Source: three-view drawing plus pictorial views. Frame: mm from the lowest corner of the part. Coordinates: 2 decimals unless noted, no trailing zeros. Write each loop counter-clockwise with the first axis right and the second up, starting at its lowest first coordinate (ties: lowest second). Pieces come first, ordered by that corner, then holes. Notation, with made-up numbers: (0.5, 70.25) - (8.5, 70.25) arc R33 ccw to (8.5, 104.25) - close; hole circle Ø7 at (-13.75, 80). An arc over 180 degrees is marked (long way). One line per item, written item: value.
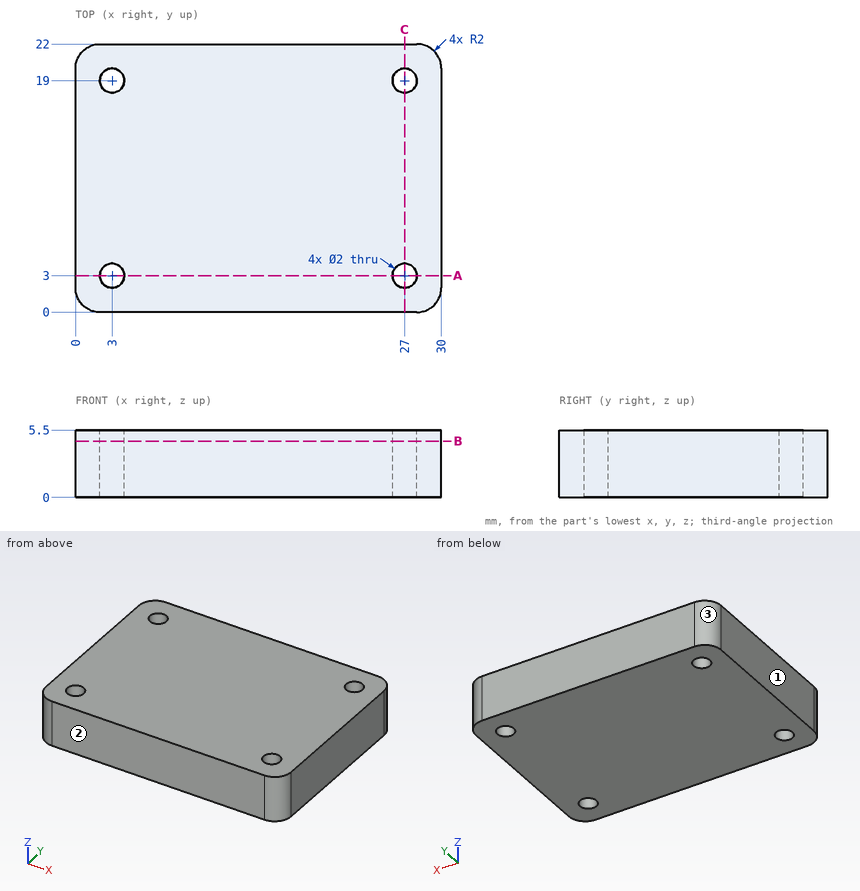
1) Section query B-B on z = 4.6. Output: boundary loops of the cut face in (x, y).
Values found:
outline: (0, 2) arc R2 ccw to (2, 0) - (28, 0) arc R2 ccw to (30, 2) - (30, 20) arc R2 ccw to (28, 22) - (2, 22) arc R2 ccw to (0, 20) - close; hole circle Ø2 at (3, 3); hole circle Ø2 at (3, 19); hole circle Ø2 at (27, 3); hole circle Ø2 at (27, 19)
2) Material intervals for line 1 (X direction, y = 3, z = 3.85); line 2 (Y direction, x = 3, z = 3.85); line 3 (Y direction, x = 2.25, z = 1.6), sorted ascending.
Values found:
line 1: 0 to 2, 4 to 26, 28 to 30
line 2: 0 to 2, 4 to 18, 20 to 22
line 3: 0 to 2.34, 3.66 to 18.34, 19.66 to 22
3) Contact query for a flat-ended pin moving along its axis: P1, Ø1.2, axis at x = 3, y = 3, coming from the -Z side. Output: stop coordinate, or through.
Values found:
P1: through
4) Section query A-A on y = 3. Output: boundary loops of the cut face in (x, z), then the cut area to 3 significant figures.
Values found:
outline: (0, 0) - (2, 0) - (2, 5.5) - (0, 5.5) - close; (4, 0) - (26, 0) - (26, 5.5) - (4, 5.5) - close; (28, 0) - (30, 0) - (30, 5.5) - (28, 5.5) - close
area: 143 mm2
5) Draft query along Y for the marked faces 1, 2 and 3. Return one class per face: released by +Y, released by -Y, zero draft, split by the parting line, or undercut.
Values found:
face 1: zero draft
face 2: released by -Y
face 3: released by +Y
6) Section query C-C on x = 27. Output: boundary loops of the cut face in (y, z).
Values found:
outline: (0, 0) - (2, 0) - (2, 5.5) - (0, 5.5) - close; (4, 0) - (18, 0) - (18, 5.5) - (4, 5.5) - close; (20, 0) - (22, 0) - (22, 5.5) - (20, 5.5) - close
